The listing builds one solid part. Answer for the finished solid, in the listing's coordinates (mm). A direction names the side the tool comes from. Give positions to 0.01 mm unless a question says otherwise; leave off trailing zeros. Write each loop counter-clockwise with the first axis right and the second up, starting at its lowest first coordinate (ties: lowest second). Pieces come first, ordered by that corner, then holes. Notation, with made-up numbers: (75.5, 3.5) -> (109.5, 3.5) arc R18 ccw to (109.5, 38.5) -> close; hole circle Ø7 at (48.5, 87). An arc over 180 degrees is marked (long way). Put each result on its own line as item: value. Start each with the question number.
1) Flat-ended cylindrical pins translate along their axes: pin 1 Ø8 at (x, z) = (-1.5, -31.5) entering from +Y (3 decimals); pin 2 Ø3 at (x, z) = (-32.5, -28.5) entering from -Y; pin 3 Ø13 at (x, y) = (-20.5, 17.5) entering from -Z; pin 4 Ø3 at (y, z) = (18.5, 6.5) entering from -X. Find the tip coordinate at first contact, or state that the pin passes through.
2) For faces 4 (the flat face through (-30, 20, 20)), 5 (the cylindrical face through (-6.014, 5.703, -16.247)), 6 (the cylindrical face through (-1.5, 36.5, 8.7)), 7 (the flat face through (-20, 20, -10)), 8 (the flat face through (-4, 0, 30)), determine the directions among +Z, -Z, +X, -X, +Y, -Y from which every point of the face is accessible in a straight line to the end or side of a thin tool.
3) Find the intervals of material crossed by line 1 along Z through (x, y) = (-18, 19.5); line 2 along X through (y, z) = (20, -21); line 3 along Y through (x, z) = (-20, -20.75), in increasing order. Write a range as from..to.
4) A cutting plane is placed at C-C (y = 36). Write down the section's boundary in (x, z), then the cut area to 3 significant figures.
5) For a pull along Y with two mould halves and no side action, classify faces 1 (the cylindrical face through (-33.986, 34.297, -0.56)), 2 (the cylindrical face through (-7.84, 16.17, -25.21)), 3 (the cylindrical face through (-33.986, 5.703, -0.56)) as released by +Y, released by -Y, zero draft, split by the parting line, or undercut.
from build123d import *

# Parameters (mm, degrees)
F1_DEPTH = 40
F2_R     = 15
F3_DEPTH = 40
F4_R     = 12.75
F5_DEPTH = 30
F6_R     = 19.99999
F7_R     = 19.99999


# Not quite as in the source:
# - a fillet or chamfer is up to 0.001 mm smaller than in the source, because OpenCascade refuses the exact size


with BuildPart() as f1:
    # F0 (on Front) → F1 (new body)
    with BuildSketch(Plane.XZ):
        Polygon((0, -40), (0, 0), (10, 0), (10, 40), (-40, 40), (-40, -40), align=None)
    extrude(amount=-F1_DEPTH)

    # F2 (on face) → F3 (cut)
    with BuildSketch(Plane.YZ.offset(10)):
        with Locations((20, 20)):
            Circle(F2_R)
    extrude(amount=-F3_DEPTH, mode=Mode.SUBTRACT)

    # F4 (on face) → F5 (cut)
    with BuildSketch(Plane(origin=(0, 0, -40), x_dir=(1, 0, 0), z_dir=(0, 0, -1))):
        with Locations((-20, -20)):
            Circle(F4_R)
    extrude(amount=-F5_DEPTH, mode=Mode.SUBTRACT)

    # F6 (radius 20 in the source; OpenCascade refuses exactly that, so slightly less here)
    f6_edges = [f1.edges().sort_by_distance(p)[0] for p in [
        (-40, 40, 0),
        (-40, 0, 0),
    ]]
    fillet(f6_edges, radius=F6_R)

    # F7 (radius 20 in the source; OpenCascade refuses exactly that, so slightly less here)
    f7_edges = [f1.edges().sort_by_distance(p)[0] for p in [
        (0, 0, -20),
        (0, 40, -20),
        (5, 0, 0),
        (5, 40, 0),
    ]]
    fillet(f7_edges, radius=F7_R)


solid = f1.part
Reply:
1. pin 1: stops at y = 33.775
1. pin 2: stops at y = 3.3
1. pin 3: stops at z = -10
1. pin 4: stops at x = -40
2. face 4: +X
2. face 5: -Z, +X, -Y
2. face 6: -Z, +X, +Y
2. face 7: -Z
2. face 8: +Z, -Z, +X, -X, -Y
3. line 1: z = -10..5.01, 34.99..40
3. line 2: x = -40..-32.75, -7.25..0
3. line 3: y = 0..7.25, 32.75..40
4. outline: (-32, -40) -> (-8, -40) -> (-8, 8) -> (10, 8) -> (10, 40) -> (-32, 40) -> close
4. area: 2,500 mm2
5. face 1: released by +Y
5. face 2: undercut
5. face 3: released by -Y
